CAD build for the part. Positions are in the model's coordinates, mm. Face numbers are marked on the shaded views. A direction names the side the tool comes from. Round coordinates to 2 decimals unless told otherwise and drop trailing zeros. Write each loop counter-clockwise with the first axis right and the second up, starting at its lowest first coordinate (ties: lowest second). Pieces come first, ordered by that corner, then holes. Notation, with made-up numbers: (41, 80.5) - (55, 80.5) arc R24 ccw to (55, 96.5) - close; hole circle Ø4 at (43, 31.5). An arc over 180 degrees is marked (long way). Use one line per item in the form item = value. Start each with the question number.
Item 1: Band-saw the part on B-B, the plane x = 24.75. List the corners of the cut face in (y, z).
Item 2: Drill centre lines: L1, parallel to Z at x = 24.75, y = 21.25; L2, parallel to X at y = 4.25, z = -15; L3, parallel to X at y = 21.25, z = 5. Where is each one in solid material? Low to high.
Item 3: Band-saw the part on D-D, the plane z = -5. List the corners of the cut face in (x, y).
Item 4: Pin check, flat tips, straight feed: pin 1 (5.5 mm diameter, centred on x = -43.75, z = 15, fed in from +Y); pin 2 (6 mm diameter, centred on x = -43, z = -4.5, fed in from +Y); pin 3 (4 mm diameter, centred on x = 15.5, y = 13.5, fed in from -Z); pin 4 (4 mm diameter, centred on y = 23, z = 3, fed in from -X). Stop position of each tip, or through.
Item 5: Pull direction Z, two halves, no side cores. Call the marked faces 1, 2 and 3: +Z half, -Z half, draft (parallel to the pull), parting line (faces both ways), or undercut.
Item 6: Band-saw the part on C-C, the plane y = 16. List the corners of the cut face in (x, z), and give its area (3 significant figures).
Item 7: Tool access for the marked faces 4, 5, 6 and 7: list every direction of +Z, -Z, +X, -X, +Y, -Y with a clear straight run to the whole face (end or side of a thin tool).
Item 8: Band-saw the part on A-A, the plane y = 7.25. List the corners of the cut face in (x, z).
from build123d import *

# Parameters (mm, degrees)
SKETCH2_W                = 20
SKETCH2_H                = 50
BOSS_EXTRUDE2_DEPTH      = 10
BOSS_EXTRUDE2_2_DEPTH    = 10
SKETCH3_W                = 7.5
SKETCH3_H                = 50
BOSS_EXTRUDE3_DEPTH      = 15
BOSS_EXTRUDE4_REACH      = 89.464
SKETCH4_W                = 50
SKETCH4_H                = 7.5
CUT_EXTRUDE1_DEPTH       = 62.23724357
CUT_EXTRUDE1_DEPTH_BACK  = 62.23724357
SKETCH6_R                = 1
SKETCH6_W                = 41
SKETCH6_H                = 21
F_6_0_6_DIAMETER_HOLE1_D = 6
SKETCH10_W               = 20
SKETCH10_H               = 10
BOSS_EXTRUDE5_DEPTH      = 17.5
CHAMFER1_SIZE            = 20


with BuildPart() as part:
    # Sketch2 → Boss-Extrude2 (new body)
    with BuildSketch(Plane(origin=(0, 0, 0), x_dir=(1, 0, 0), z_dir=(0, 1, 0))):
        with Locations((-40, 0)):
            Rectangle(SKETCH2_W, SKETCH2_H)
    extrude(amount=BOSS_EXTRUDE2_DEPTH)



with BuildPart() as body_2:
    # Sketch2 → Boss-Extrude2 2 (new body)
    with BuildSketch(Plane(origin=(0, 0, 0), x_dir=(1, 0, 0), z_dir=(0, 1, 0))):
        with Locations((40, 0)):
            Rectangle(SKETCH2_W, SKETCH2_H)
    extrude(amount=BOSS_EXTRUDE2_2_DEPTH)


with BuildPart() as part_1:
    add(part.part)

    add(body_2.part)  # Boss-Extrude3 merges body 2
    # Sketch3 → Boss-Extrude3 (add)
    with BuildSketch(Plane(origin=(0, 10, 0), x_dir=(1, 0, 0), z_dir=(0, 1, 0))):
        with Locations((-33.75, 0)):
            Rectangle(SKETCH3_W, SKETCH3_H)
        with Locations((33.75, 0)):
            Rectangle(SKETCH3_W, SKETCH3_H)
    extrude(amount=BOSS_EXTRUDE3_DEPTH)

    # Sketch4 → Boss-Extrude4 (add, up to next)
    with BuildSketch(Plane.ZY.offset(-30), mode=Mode.PRIVATE) as boss_extrude4_sk1:
        with Locations((0, 21.25)):
            Rectangle(SKETCH4_W, SKETCH4_H)
    boss_extrude4_tool1 = extrude(boss_extrude4_sk1.sketch, amount=BOSS_EXTRUDE4_REACH, mode=Mode.PRIVATE) - part_1.part
    add(boss_extrude4_tool1.solids().sort_by_distance((30, 21.25, 0))[0])

    # Sketch6 → Cut-Extrude1 (cut, two sides: drawn at the far end of the back side and taken through both)
    with BuildSketch(Plane(origin=(0, 25, 0), x_dir=(1, 0, 0), z_dir=(0, 1, 0)).offset(-CUT_EXTRUDE1_DEPTH_BACK)):
        with Locations(Location((24.75, 5, 0), (0, 0, 270))):
            Circle(SKETCH6_R)
        with Locations(Location((24.75, -5, 0), (0, 0, 270))):
            Circle(SKETCH6_R)
        with Locations(Location((-24.75, 5, 0), (0, 0, 270))):
            Circle(SKETCH6_R)
        with Locations(Location((-24.75, -5, 0), (0, 0, 270))):
            Circle(SKETCH6_R)
        Rectangle(SKETCH6_W, SKETCH6_H)
    extrude(amount=CUT_EXTRUDE1_DEPTH + CUT_EXTRUDE1_DEPTH_BACK, mode=Mode.SUBTRACT)

    # Ø6.0 (6) Diameter Hole1 (through all)
    with Locations(Plane(origin=(-43.75, 10, -15), x_dir=(0, 0, 1), z_dir=(0, 1, 0))):
        with Locations((0, 0), (30, 0), (30, 87.5), (0, 87.5)):
            Hole(F_6_0_6_DIAMETER_HOLE1_D / 2)

    # Sketch10 → Boss-Extrude5 (add)
    with BuildSketch(Plane.XZ.offset(-17.5)):
        with Locations((-20, 20)):
            Rectangle(SKETCH10_W, SKETCH10_H)
        with Locations((20, 20)):
            Rectangle(SKETCH10_W, SKETCH10_H)
    extrude(amount=BOSS_EXTRUDE5_DEPTH)

    # Chamfer1
    # the kernel refuses this chamfer: 20 mm, written as the material it adds along each edge
    # the kernel refuses this chamfer: 20 mm, written as the material it takes off along each edge
    with BuildSketch(Plane(origin=(10, 0, 76.433659759), x_dir=(0.9996219169112968, -0.027495876610586372, 0), z_dir=(0, 0, -1))) as chamfer1_2_piece_1_section:
        Polygon((CHAMFER1_SIZE * 0.999621916911, -CHAMFER1_SIZE * 0.0274958766106), (-CHAMFER1_SIZE * 0.0274958766106, -CHAMFER1_SIZE * 0.999621916911), (0, 0), align=None)
    chamfer1_2_piece_1 = extrude(amount=112.867319519, mode=Mode.PRIVATE)
    chamfer1_2_piece_1 = split(chamfer1_2_piece_1, bisect_by=Plane(origin=(16.759259259, 17.5, 20), z_dir=(0, -1, 0)), keep=Keep.TOP, mode=Mode.PRIVATE)
    add(chamfer1_2_piece_1, mode=Mode.SUBTRACT)
    with BuildSketch(Plane(origin=(-10, 0, 76.433659759), x_dir=(0.027495876610586403, 0.9996219169112968, 0), z_dir=(0, 0, -1))) as chamfer1_2_piece_2_section:
        Polygon((CHAMFER1_SIZE * 0.999621916911, -CHAMFER1_SIZE * 0.0274958766106), (-CHAMFER1_SIZE * 0.0274958766106, -CHAMFER1_SIZE * 0.999621916911), (0, 0), align=None)
    chamfer1_2_piece_2 = extrude(amount=112.867319519, mode=Mode.PRIVATE)
    chamfer1_2_piece_2 = split(chamfer1_2_piece_2, bisect_by=Plane(origin=(-16.759259259, 17.5, 20), z_dir=(0, -1, 0)), keep=Keep.TOP, mode=Mode.PRIVATE)
    add(chamfer1_2_piece_2, mode=Mode.SUBTRACT)


solid = part_1.part
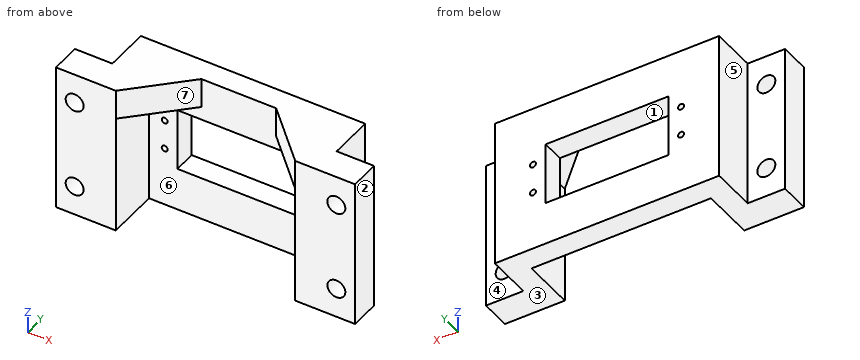
Determined:
q1.outline = (5.25, 15) - (17.5, 15) - (17.5, 6) - (25, 6) - (25, 25) - (5.25, 25) - close; (17.5, -25) - (25, -25) - (25, -6) - (17.5, -6) - close; (17.5, -4) - (25, -4) - (25, 4) - (17.5, 4) - close
q2.L1 = -25 to -6, -4 to 4, 6 to 25
q2.L2 = -50 to -46.75, -40.75 to -30, 30 to 40.75, 46.75 to 50
q2.L3 = -37.5 to -25.75, -23.75 to -20.5, 20.5 to 23.75, 25.75 to 37.5
q3.outline = (-50, 0) - (-30, 0) - (-30, 17.5) - (-25.75, 17.5) - (-25.75, 25) - (-37.5, 25) - (-37.5, 10) - (-50, 10) - close; (-23.75, 17.5) - (-20.5, 17.5) - (-20.5, 25) - (-23.75, 25) - close; (20.5, 17.5) - (23.75, 17.5) - (23.75, 25) - (20.5, 25) - close; (25.75, 17.5) - (30, 17.5) - (30, 0) - (50, 0) - (50, 10) - (37.5, 10) - (37.5, 25) - (25.75, 25) - close
q4.pin_1 = through
q4.pin_2 = 10
q4.pin_3 = 15
q4.pin_4 = -37.5
q5.face_1 = undercut
q5.face_2 = draft
q5.face_3 = -Z half
q6.outline = (-37.5, -25) - (-30, -25) - (-30, 15) - (-14, 15) - (-14, 25) - (-37.5, 25) - close; (14, 15) - (30, 15) - (30, -25) - (37.5, -25) - (37.5, 25) - (14, 25) - close
q6.area = 1,070 mm²
q7.face_4 = +Z, -Z, +X, +Y
q7.face_5 = +Z, -Z, -X, +Y
q7.face_6 = -Z, -Y
q7.face_7 = +Z, -Z, -Y
q8.outline = (-50, -25) - (-30, -25) - (-30, 15) - (-22.75, 15) - (-22.75, 25) - (-50, 25) - close; (22.75, 15) - (30, 15) - (30, -25) - (50, -25) - (50, 25) - (22.75, 25) - close; hole circle Ø6 at (-43.75, -15); hole circle Ø6 at (-43.75, 15); hole circle Ø6 at (43.75, -15); hole circle Ø6 at (43.75, 15)
